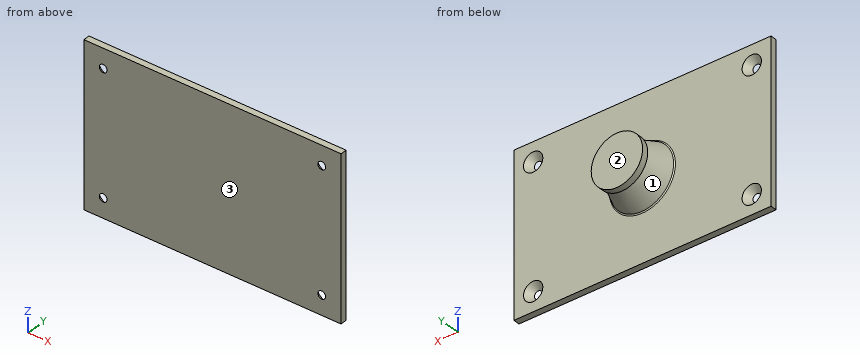
from build123d import *

# Parameters (mm, degrees)
SKETCH1_W                = 50.8
SKETCH1_H                = 31.75
BOSS_EXTRUDE1_DEPTH      = 1.27
BOSS_EXTRUDE2_DEPTH      = 6.35
BOSS_EXTRUDE2_DEPTH_BACK = 1.27
SKETCH2_R                = 6.35
CHAMFER1_SIZE            = 6.35
CHAMFER1_SIZE_2          = 2.54
FILLET1_R                = 0.254
SKETCH7_R                = 5.08
BOSS_EXTRUDE3_DEPTH      = 1.27


with BuildPart() as part:
    # Sketch1 → Boss-Extrude1 (new body)
    with BuildSketch(Plane(origin=(0, 0, 0), x_dir=(1, 0, 0), z_dir=(0, 1, 0))):
        Rectangle(SKETCH1_W, SKETCH1_H)
    extrude(amount=BOSS_EXTRUDE1_DEPTH)

    # Sketch2 → Boss-Extrude2 (add, two sides: drawn at the far end of the back side and taken through both)
    with BuildSketch(Plane(origin=(0, 1.27, 0), x_dir=(1, 0, 0), z_dir=(0, 1, 0)).offset(-BOSS_EXTRUDE2_DEPTH_BACK)):
        with Locations(Location((0, 0, 0), (0, 0, 270))):
            Circle(SKETCH2_R)
    extrude(amount=BOSS_EXTRUDE2_DEPTH + BOSS_EXTRUDE2_DEPTH_BACK)

    # Chamfer1
    # the kernel refuses this chamfer: 6.35, 2.54 mm, written as the material it takes off along each edge
    with BuildSketch(Plane(origin=(0, 7.62, 0), x_dir=(0, 0, 1), z_dir=(-1, 0, 0))) as chamfer1_piece_1_section:
        Polygon((6.35, -CHAMFER1_SIZE), (6.35 - CHAMFER1_SIZE_2, 0), (6.35, 0), align=None)
    chamfer1_piece_1 = revolve(axis=Axis((0, 7.62, 0), (0, 1, 0)), mode=Mode.PRIVATE)
    chamfer1_piece_1 = split(chamfer1_piece_1, bisect_by=Plane(origin=(0, 1.27, -5.09685111), z_dir=(0, 1, 0)), keep=Keep.TOP, mode=Mode.PRIVATE)
    add(chamfer1_piece_1, mode=Mode.SUBTRACT)

    # Fillet1
    fillet1_edges = [part.edges().sort_by_distance(p)[0] for p in [
        (0, 1.27, -6.35),
    ]]
    fillet(fillet1_edges, radius=FILLET1_R)

    # Sketch6 → Cut-Revolve1 (revolve, cut)
    with BuildSketch(Plane.XY.offset(12.065), mode=Mode.PRIVATE) as cut_revolve1_sk:
        Polygon((21.59, 1.27), (21.59, 0), (20.828, 0), (19.685, 1.27), align=None)
    cut_revolve1 = revolve(cut_revolve1_sk.sketch.rotate(Axis((21.59, 1.27, 12.065), (0, -1, 0)), 270), axis=Axis((21.59, 1.27, 12.065), (0, -1, 0)), mode=Mode.SUBTRACT)

    # Mirror1: Cut-Revolve1 across plane
    add(cut_revolve1.mirror(Plane.XY), mode=Mode.SUBTRACT)

    # Mirror2: Cut-Revolve1 across plane
    add(cut_revolve1.mirror(Plane(origin=(0, 0, 0), x_dir=(0, 0, 1), z_dir=(1, 0, 0))), mode=Mode.SUBTRACT)

    # Mirror2 copy 1 sketch → Mirror2 copy 1 (revolve, cut)
    with BuildSketch(Plane(origin=(0, 0, -12.065), x_dir=(-1, 0, 0), z_dir=(0, 0, -1))):
        Polygon((21.59, 1.27), (21.59, 0), (20.828, 0), (19.685, 1.27), align=None)
    revolve(axis=Axis((-21.59, 1.27, -12.065), (0, -1, 0)), mode=Mode.SUBTRACT)

    # Sketch7 → Boss-Extrude3 (add)
    with BuildSketch(Plane(origin=(0, 7.62, 0), x_dir=(1, 0, 0), z_dir=(0, 1, 0))):
        with Locations(Location((0, 0, 0), (0, 0, 270))):
            Circle(SKETCH7_R)
    extrude(amount=-BOSS_EXTRUDE3_DEPTH)


solid = part.part
Design review of the part built by this model. Coordinates are the model's own, in mm. Face numbers are marked on the shaded views. Round coordinates to 2 decimals unless told otherwise and drop trailing zeros. Loops run counter-clockwise (first coordinate to the right, second up) from the corner with the lowest first, then second, coordinate; pieces in that order, holes last. Notation, with made-up numbers: (-25.5, 85.5) - (10.5, 85.5) arc R17 ccw to (10.5, 117.5) - close; hole circle Ø6 at (36.25, 12.25). An arc over 180 degrees is marked (long way). One line per item, written item: value. Start each with the question number.
1) Consider section B-B on x = 0. Give the boundary of the cut face in (y, z) (3 decimals).
2) To check wall thickness, follow L1, parallel to Y at x = -6, z = 7; L2, parallel to Y at x = -4.5, z = -2; L3, parallel to X at y = 5.5, z = -0.5. State the ranges of each line that lie inside material, in increasing order. Write a range as from..to.
3) Insertion check: pin 1 Ø3 at (y, z) = (1.5, 0.5) entering from +X; pin 2 Ø1.5 at (y, z) = (5.5, 3.5) entering from -X; pin 3 Ø1.5 at (x, y) = (14.5, 3.5) entering from -Z. Each pin has a flat end and moves straight along its axis. Give the tip position at first contact, or say it passes through.
4) Consider section A-A on x = 21.59. Give the boundary of the cut face in (y, z) (3 decimals).
5) Draft analysis for pull direction Y (two halves, no side actions). For the marked faces 1, 2 and 3, state which applies: +Y half, -Y half, draft (parallel to the pull), parting line (faces both ways), or undercut.
6) Consider section D-D on y = 4.25. Give the boundary of the cut face in (x, z).
7) Consider section C-C on z = 0. Give the boundary of the cut face in (x, y), then the cut area to 3 significant figures.
Reported:
1. outline: (0, -15.875) - (1.27, -15.875) - (1.27, -6.522) arc R0.254 cw to (1.43, -6.286) - (6.35, -4.318) - (6.35, -5.08) - (7.62, -5.08) - (7.62, 5.08) - (6.35, 5.08) - (6.35, 4.318) - (1.43, 6.286) arc R0.254 cw to (1.27, 6.522) - (1.27, 15.875) - (0, 15.875) - close
2. L1: y = 0..1.27
2. L2: y = 0..4.83, 6.35..7.62
2. L3: x = -4.63..4.63
3. pin 1: stops at x = 25.4
3. pin 2: stops at x = -3.87
3. pin 3: passes through
4. outline: (0, -15.875) - (1.27, -15.875) - (1.27, -13.97) - (0, -12.827) - close; (0, -11.303) - (1.27, -10.16) - (1.27, 10.16) - (0, 11.303) - close; (0, 12.827) - (1.27, 13.97) - (1.27, 15.875) - (0, 15.875) - close
5. face 1: undercut
5. face 2: +Y half
5. face 3: -Y half
6. outline: circle Ø10.32 at (0, 0)
7. outline: (-25.4, 0) - (25.4, 0) - (25.4, 1.27) - (6.52, 1.27) arc R0.25 cw to (6.29, 1.43) - (4.32, 6.35) - (5.08, 6.35) - (5.08, 7.62) - (-5.08, 7.62) - (-5.08, 6.35) - (-4.32, 6.35) - (-6.29, 1.43) arc R0.25 cw to (-6.52, 1.27) - (-25.4, 1.27) - close
7. area: 132 mm^2
